from build123d import *

# Parameters (mm, degrees)
F1_DEPTH  = 2.4
F2_W      = 1
F2_H      = 15
F3_DEPTH  = 12.5
F5_W      = 2.8
F5_H      = 0.8
F6_DEPTH  = 0.8
F8_DEPTH  = 2.401
F9_R      = 1.3
F10_DEPTH = 2.401


with BuildPart() as f1:
    # F0 (on Front) → F1 (new body)
    with BuildSketch(Plane.XZ):
        with BuildLine():
            Line((-7.5, 4.37), (-7.5, -6.229968))
            ThreePointArc((-7.5, -6.229968), (-6.316015, -7.427682), (-4.943581, -8.403779))
            Line((-4.943581, -8.403779), (4.943581, -8.403779))
            ThreePointArc((4.943581, -8.403779), (6.316015, -7.427682), (7.5, -6.229968))
            Line((7.5, -6.229968), (7.5, 4.37))
            Line((7.5, 4.37), (10.907135, 4.37))
            ThreePointArc((10.907135, 4.37), (0, 11.75), (-10.907135, 4.37))
            Line((-10.907135, 4.37), (-7.5, 4.37))
        make_face()
    extrude(amount=F1_DEPTH)

    # F2 (on Right) → F3 (cut, symmetric)
    with BuildSketch(Plane.YZ):
        with Locations((-0.5, -3.13)):
            Rectangle(F2_W, F2_H)
    extrude(amount=F3_DEPTH, both=True, mode=Mode.SUBTRACT)

    # F5 (on offset) → F6 (cut)
    with BuildSketch(Plane.XY.offset(12)):
        with Locations((0, -1.2)):
            Rectangle(F5_W, F5_H)
    extrude(amount=-F6_DEPTH, mode=Mode.SUBTRACT)

    # F7 (on face) → F8 (cut, through all)
    with BuildSketch(Plane.XZ.offset(2.4)):
        with BuildLine():
            Line((-3.195484, 7.75), (-3.195484, 11.307139))
            ThreePointArc((-3.195484, 11.307139), (-6.271121, 9.936576), (-8.831761, 7.75))
            Line((-8.831761, 7.75), (-3.195484, 7.75))
        make_face()
        with BuildLine():
            Line((3.195484, 7.75), (8.831761, 7.75))
            ThreePointArc((8.831761, 7.75), (6.271121, 9.936576), (3.195484, 11.307139))
            Line((3.195484, 11.307139), (3.195484, 7.75))
        make_face()
    extrude(amount=-F8_DEPTH, mode=Mode.SUBTRACT)

    # F9 (on face) → F10 (cut, through all)
    with BuildSketch(Plane.XZ.offset(2.4)):
        Circle(F9_R)
    extrude(amount=-F10_DEPTH, mode=Mode.SUBTRACT)


solid = f1.part
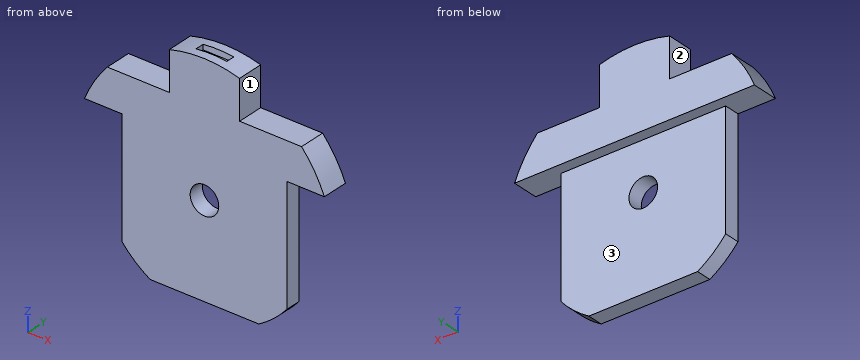
Part model, mm, in its own coordinate system. Face numbers are marked on the shaded views. A direction names the side the tool comes from. Give positions to 0.01 mm unless a question says otherwise; leave off trailing zeros. Loops run counter-clockwise (first coordinate to the right, second up) from the corner with the lowest first, then second, coordinate; pieces in that order, holes last.
(1) Band-saw the part on C-C (y = -1.95). Write the cut outline in (x, z).
Return value:
outline: (-10.91, 4.37) - (-7.5, 4.37) - (-7.5, -6.23) arc R9.75 ccw to (-4.94, -8.4) - (4.94, -8.4) arc R9.75 ccw to (7.5, -6.23) - (7.5, 4.37) - (10.91, 4.37) arc R11.75 ccw to (8.83, 7.75) - (3.2, 7.75) - (3.2, 11.31) arc R11.75 ccw to (-3.2, 11.31) - (-3.2, 7.75) - (-8.83, 7.75) arc R11.75 ccw to start; hole circle Ø2.6 at (0, 0)
(2) Band-saw the part on A-A (z = 0). Write the cut outline in (x, y).
Return value:
outline: (-7.5, -2.4) - (-1.3, -2.4) - (-1.3, -1) - (-7.5, -1) - close; (1.3, -2.4) - (7.5, -2.4) - (7.5, -1) - (1.3, -1) - close
(3) Drill centre lines: line 1 along Z through (x, y) = (0, -1.95); line 2 along X through (y, z) = (-1.35, -3.5); line 3 along Y through (x, z) = (-1.5, -1.5). Where is each one in solid material? Low to high.
Return value:
line 1: z = -8.4 to -1.3, 1.3 to 11.75
line 2: x = -7.5 to 7.5
line 3: y = -2.4 to -1
(4) Band-saw the part on D-D (x = -4.5). Write the cut outline in (y, z), and give its area (3 significant figures).
Return value:
outline: (-2.4, -8.4) - (-1, -8.4) - (-1, 4.37) - (0, 4.37) - (0, 7.75) - (-2.4, 7.75) - close
area: 26.0 mm2
(5) Pin check, flat tips, straight feed: pin 1 (2 mm diameter, centred on x = 0, z = 0, fed in from -Y); pin 2 (1.1 mm diameter, centred on y = -2, z = -1, fed in from +X); pin 3 (0.7 mm diameter, centred on y = -1, z = 10, fed in from +X); pin 4 (6.5 mm diameter, centred on x = 1, z = 0, fed in from +Y). Stop position of each tip, or through.
Return value:
pin 1: passes through
pin 2: stops at x = 7.5
pin 3: stops at x = 3.2
pin 4: stops at y = -1
(6) Band-saw the part on B-B (x = 0). Write the cut outline in (y, z), and give its area (3 significant figures).
Return value:
outline: (-2.4, -8.4) - (-1, -8.4) - (-1, -1.3) - (-2.4, -1.3) - close; (-2.4, 1.3) - (-1, 1.3) - (-1, 4.37) - (0, 4.37) - (0, 11.75) - (-0.8, 11.75) - (-0.8, 11.2) - (-1.6, 11.2) - (-1.6, 11.75) - (-2.4, 11.75) - close
area: 31.5 mm2
(7) 3-axis set-ups, long thin cutter, end or side, ignore diameter. For the marked faces 1, 2 and 3: which of +Z, -Z, +X, -X, +Y, -Y reach the whole face in a straight line?
Return value:
face 1: +Z, +X, +Y, -Y
face 2: +Z, -X, +Y, -Y
face 3: -Z, +X, -X, +Y
